Read the model definition and answer for the solid it produces. Units are mm, in the model's axes. A direction names the side the tool comes from. Give positions to 0.01 mm unless a question says otherwise; leave off trailing zeros. Loops run counter-clockwise (first coordinate to the right, second up) from the corner with the lowest first, then second, coordinate; pieces in that order, holes last. Notation, with made-up numbers: M -14,75.5 L 20,75.5 A26 ccw 20,102.5 Z; hole C 34,-8 d6. An arc over 180 degrees is marked long. Return JSON: item names as keys, results as strings. Group by question number.
```python
from build123d import *

# Parameters (mm, degrees)
F0_W     = 80
F0_H     = 1650
F1_DEPTH = 40
F2_W     = 80
F2_H     = 40
F3_DEPTH = 800
F5_DEPTH = 40


with BuildPart() as f1:
    # F0 (on Right) → F1 (new body)
    with BuildSketch(Plane.YZ):
        with Locations((40, 825)):
            Rectangle(F0_W, F0_H)
    extrude(amount=-F1_DEPTH)

    # F2 (on face) → F3 (join)
    with BuildSketch(Plane(origin=(-40, 0, 0), x_dir=(0, -1, 0), z_dir=(-1, 0, 0))):
        with Locations((-40, 1062)):
            Rectangle(F2_W, F2_H)
    extrude(amount=F3_DEPTH)

    # F4 (on face) → F5 (join)
    with BuildSketch(Plane(origin=(0, 0, 1042), x_dir=(1, 0, 0), z_dir=(0, 0, -1))):
        Polygon((-40, -820), (-40, 830), (-120, 830), (-120, -740), (-425, -740), (-425, 830), (-505, 830), (-505, -820), align=None)
    extrude(amount=F5_DEPTH)


solid = f1.part
```
1. Find section B-B (y = 674.5). Write down the section's boundary in (x, z), and give its area (3 significant figures).
2. Find section D-D (x = -82.5). Write down the section's boundary in (y, z), and give its area (3 significant figures).
3. Flat-ended cylindrical pins translate along their axes: P1, Ø12, axis at y = -382.5, z = 1028.5, coming from the -X side; P2, Ø12, axis at y = 340.5, z = 1021, coming from the +X side. Find the tip coordinate at first contact, or state that the pin passes through.
4. Find section C-C (z = 319.5). Write down the section's boundary in (x, y), and give its area (3 significant figures).
5. For faces 1 (the flat face through (-40, 455, 1022)), 2 (the flat face through (-270, 740, 1022)), 3 (the flat face through (-81, -421, 1042)), 4 (the flat face through (-670, 41, 1042)), 5 (the flat face through (-431, 527, 1042)), determine the directions among +Z, -Z, +X, -X, +Y, -Y from which every point of the face is accessible in a straight line to the end or side of a thin tool.
6. Straight lines are drawn through the part: line 1 along Z through (x, y) = (-461.5, 171.5); line 2 along Z through (x, y) = (-493, 44). For each, find the intervals that lie inside material, in ascending order.
7. The mould has two halves that part along X. Classify faces 6 (the flat face through (-466, -421, 1042)), 7 (the flat face through (-425, -34, 1022)), 8 (the flat face through (-270, 41, 1042)), 9 (the flat face through (-40, 39, 1370)): +X half, -X half, draft (parallel to the pull), parting line (faces both ways), or undercut.
8. Find section A-A (x = -225). Write down the section's boundary in (y, z), and give its area (3 significant figures).
Result:
{
 "1": {"outline": "M -505,1002 L -425,1002 L -425,1042 L -505,1042 Z; M -120,1002 L -40,1002 L -40,1042 L -120,1042 Z", "area": "6,400 mm2"},
 "2": {"outline": "M -830,1002 L 820,1002 L 820,1042 L 80,1042 L 80,1082 L 0,1082 L 0,1042 L -830,1042 Z", "area": "69,200 mm2"},
 "3": {"P1": "stops at x = -505", "P2": "stops at x = -40"},
 "4": {"outline": "M -40,0 L 0,0 L 0,80 L -40,80 Z", "area": "3,200 mm2"},
 "5": {"face 1": "+Z, -Z, +X, +Y", "face 2": "+Z, -Z, -Y", "face 3": "+Z, +X, -X, -Y", "face 4": "-Z, -X, +Y, -Y", "face 5": "+Z, +X, -X, +Y"},
 "6": {"line 1": "z = 1002 to 1042", "line 2": "z = 1002 to 1082"},
 "7": {"face 6": "draft", "face 7": "undercut", "face 8": "undercut", "face 9": "-X half"},
 "8": {"outline": "M 0,1042 L 80,1042 L 80,1082 L 0,1082 Z; M 740,1002 L 820,1002 L 820,1042 L 740,1042 Z", "area": "6,400 mm2"}
}
